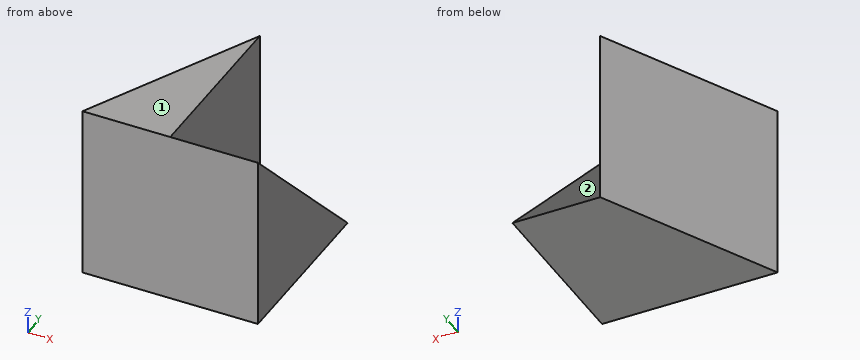
from build123d import *

# Parameters (mm, degrees)
SKETCH1_W           = 40
SKETCH1_H           = 40
BOSS_EXTRUDE1_DEPTH = 40
CUT_EXTRUDE1_DEPTH  = 40
CUT_EXTRUDE3_DEPTH  = 20


with BuildPart() as part:
    # Sketch1 → Boss-Extrude1 (new body)
    with BuildSketch(Plane.XY):
        with Locations((20, 20)):
            Rectangle(SKETCH1_W, SKETCH1_H)
    extrude(amount=BOSS_EXTRUDE1_DEPTH)

    # Sketch2 → Cut-Extrude1 (cut)
    with BuildSketch(Plane.XY.offset(40)):
        Polygon((0, 0), (20, 40), (0, 40), align=None)
    extrude(amount=-CUT_EXTRUDE1_DEPTH, mode=Mode.SUBTRACT)

    # Sketch3 → Cut-Extrude3 (cut)
    with BuildSketch(Plane(origin=(40, 0, 0), x_dir=(0, 0, -1), z_dir=(1, 0, 0))):
        Polygon((0, 40), (-40, 40), (-20, 20), align=None)
        Polygon((-20, 20), (-40, 40), (-40, 0), align=None)
    extrude(amount=-CUT_EXTRUDE3_DEPTH, mode=Mode.SUBTRACT)


solid = part.part
For this review, take the finished solid that the model builds, in its own axes (mm). Face numbers are marked on the shaded views. A direction names the side the tool comes from. Round coordinates to 2 decimals unless told otherwise and drop trailing zeros. Loops run counter-clockwise (first coordinate to the right, second up) from the corner with the lowest first, then second, coordinate; pieces in that order, holes last. Notation, with made-up numbers: (73.5, 57.5) - (106.5, 57.5) arc R14 ccw to (106.5, 84.5) - close; hole circle Ø7 at (-14.75, 67). An arc over 180 degrees is marked (long way). One line per item, written item: value. Start each with the question number.
Item 1: Take a section at B-B (z = 36). Give the boundary of the cut face in (x, y).
Item 2: Take a section at A-A (y = 29). Give the boundary of the cut face in (x, z), plus the area to 3 significant figures.
Item 3: Clearance check with flat-ended pins moving along their axes: pin 1 Ø2 at (x, z) = (28.5, 21.5) entering from +Y; pin 2 Ø2 at (x, z) = (29, 6) entering from +Y; pin 3 Ø6 at (x, z) = (5, 33) entering from +Y. State where each tip first meets the part, or that it passes through.
Item 4: Take a section at C-C (x = 14). Give the boundary of the cut face in (y, z), plus the area to 3 significant figures.
Item 5: For the marked faces 1 and 2, list the 3-axis set-ups (+Z, -Z, +X, -X, +Y, -Y) from which the entire face can be reached by the end or side of a thin tool; tool diameter is ignored.
Item 6: Take a section at D-D (z = 17). Give the boundary of the cut face in (x, y), plus the area to 3 significant figures.
Item 7: For L1, parallel to X at y = 9, z = 27; L2, parallel to Y at x = 19, z = 18; L3, parallel to Y at x = 33, z = 16.5, list the stretches that pass through material, from the lowest coordinate up.
Answer below:
1. outline: (0, 0) - (40, 0) - (40, 4) - (20, 4) - (20, 40) - close
2. outline: (14.5, 0) - (40, 0) - (40, 11) - (20, 11) - (20, 40) - (14.5, 40) - close
2. area: 440 mm2
3. pin 1: stops at y = 19.5
3. pin 2: stops at y = 35
3. pin 3: stops at y = 16
4. outline: (0, 0) - (28, 0) - (28, 40) - (0, 40) - close
4. area: 1,120 mm2
5. face 1: +Z, +X, -X, +Y, -Y
5. face 2: +Z, +X, +Y
6. outline: (0, 0) - (40, 0) - (40, 23) - (20, 23) - (20, 40) - close
6. area: 860 mm2
7. L1: x = 4.5 to 40
7. L2: y = 0 to 38
7. L3: y = 0 to 23.5
